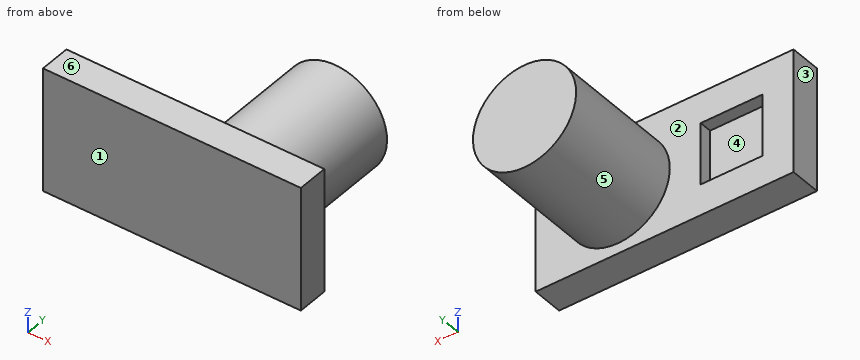
```python
from build123d import *

# Parameters (mm, degrees)
SKETCH1_W          = 125
SKETCH1_H          = 60
EXTRUDE1_DEPTH     = 15
SKETCH2_R          = 25
EXTRUDE2_DEPTH     = 60
SKETCH3_W          = 30
SKETCH3_H          = 30
CUT_EXTRUDE1_DEPTH = 6


with BuildPart() as part:
    # Sketch1 → Extrude1 (new body)
    with BuildSketch(Plane(origin=(0, 0, 0), x_dir=(1, 0, 0), z_dir=(0, 1, 0))):
        with Locations((62.5, 30)):
            Rectangle(SKETCH1_W, SKETCH1_H)
    extrude(amount=EXTRUDE1_DEPTH)

    # Sketch2 → Extrude2 (add)
    with BuildSketch(Plane(origin=(0, 15, 0), x_dir=(-1, 0, 0), z_dir=(0, 1, 0))):
        with Locations(Location((-85, -30, 0), (0, 0, 270))):  # turned: the seam where the file's is
            Circle(SKETCH2_R)
    extrude(amount=EXTRUDE2_DEPTH)

    # Sketch3 → Cut-Extrude1 (cut)
    with BuildSketch(Plane(origin=(0, 15, 0), x_dir=(-1, 0, 0), z_dir=(0, 1, 0))):
        with Locations((-30, -30)):
            Rectangle(SKETCH3_W, SKETCH3_H)
    extrude(amount=-CUT_EXTRUDE1_DEPTH, mode=Mode.SUBTRACT)


solid = part.part
```
Input: part model. Units: mm. Frame: model coordinates. Face numbers are marked on the shaded views. A direction names the side the tool comes from. Coordinates: 2 decimals unless noted, no trailing zeros. Loops run counter-clockwise (first coordinate to the right, second up) from the corner with the lowest first, then second, coordinate; pieces in that order, holes last.
Q1. Section A-A, the plane x = 36. Return the cut outline in (y, z).
Results are:
outline: (0, -60) - (15, -60) - (15, -45) - (9, -45) - (9, -15) - (15, -15) - (15, 0) - (0, 0) - close
Q2. Section B-B, the plane z = -30. Return the cut outline in (x, y).
Results are:
outline: (0, 0) - (125, 0) - (125, 15) - (110, 15) - (110, 75) - (60, 75) - (60, 15) - (45, 15) - (45, 9) - (15, 9) - (15, 15) - (0, 15) - close
Q3. Section C-C, the plane y = 51. Return the cut outline in (x, z).
Results are:
outline: circle Ø50 at (85, -30)
Q4. Mould query, pull axis X, two halves, no side actions, for the marked faces 3, 4, 5 and 6. Classes: +X half, -X half, draft (parallel to the pull), parting line (faces both ways), or undercut.
Results are:
face 3: -X half
face 4: undercut
face 5: parting line
face 6: draft
Q5. Section D-D, the plane x = 85. Return the cut outline in (y, z).
Results are:
outline: (0, -60) - (15, -60) - (15, -55) - (75, -55) - (75, -5) - (15, -5) - (15, 0) - (0, 0) - close
Q6. Set-up query: the marked faces 1 and 2. Return all of +Z, -Z, +X, -X, +Y, -Y with unobstructed straight access to the full face (end or side cutting, diameter ignored); none if empty.
Results are:
face 1: +Z, -Z, +X, -X, -Y
face 2: +Y
Q7. Contact query for flat-ended pins moving along their axis: pin 1 (1 mm diameter, centred on x = 71, y = 43, fed in from -Z); pin 2 (3 mm diameter, centred on x = 69, y = 40.5, fed in from -Z); pin 3 (3 mm diameter, centred on x = 66, y = 28, fed in from -Z). Output: stop coordinate, or through.
Results are:
pin 1: stops at z = -51.04
pin 2: stops at z = -50.37
pin 3: stops at z = -47.85
Q8. Line query: line 1 along Z through (x, y) = (34.5, 11.5); line 2 along X through (y, z) = (9.5, -33.5); line 3 along Y through (x, z) = (37.5, -42). Output: solid intervals per line, ascending.
Results are:
line 1: z = -60 to -45, -15 to 0
line 2: x = 0 to 15, 45 to 125
line 3: y = 0 to 9
